from build123d import *

# Parameters (mm, degrees)
BOSS_EXTRUDE1_DEPTH = 40
FILLET1_R           = 0.5


with BuildPart() as part:
    # Sketch1 → Boss-Extrude1 (new body)
    with BuildSketch(Plane(origin=(0, 0, 0), x_dir=(-1, 0, 0), z_dir=(0, 1, 0))):
        with BuildLine():
            Line((-16.382358243, -12.416132382), (-16.309116245, 1.980717277))
            Line((-16.309116245, 1.980717277), (-2.623220974, -2.488165706))
            ThreePointArc((-2.623220974, -2.488165706), (-1.953288331, -2.586352132), (-1.288986221, -2.455382561))
            Line((-1.288986221, -2.455382561), (11.279166812, 2.343564434))
            Line((11.279166812, 2.343564434), (11.764255017, -12.063312843))
            ThreePointArc((11.764255017, -12.063312843), (11.874027832, -12.652761031), (12.15358265, -13.183183826))
            Line((12.15358265, -13.183183826), (20.699476347, -24.769483728))
            Line((20.699476347, -24.769483728), (7.033191834, -29.354905309))
            ThreePointArc((7.033191834, -29.354905309), (6.499122182, -29.629147424), (6.070505236, -30.049536105))
            Line((6.070505236, -30.049536105), (-2.58921338, -41.573541353))
            Line((-2.58921338, -41.573541353), (-10.890805488, -29.810964554))
            ThreePointArc((-10.890805488, -29.810964554), (-11.306058502, -29.378455396), (-11.830848647, -29.088464807))
            Line((-11.830848647, -29.088464807), (-25.350255054, -24.086557786))
            Line((-25.350255054, -24.086557786), (-16.834067363, -13.67200498))
            ThreePointArc((-16.834067363, -13.67200498), (-16.500364189, -13.082859401), (-16.382358243, -12.416132382))
        make_face()
    extrude(amount=BOSS_EXTRUDE1_DEPTH)

    # Fillet1
    fillet1_edges = [part.edges().sort_by_distance(p)[0] for p in [
        (18.59055185, 40, -26.587511297),
        (16.345737244, 0, -5.217707553),
        (9.46616861, 0, -0.253724215),
        (1.953288331, 0, -2.586352132),
        (-4.995090296, 0, -0.055909063),
        (-11.521710915, 0, -4.859874204),
        (-11.874027832, 0, -12.652761031),
        (11.306058502, 40, -29.378455396),
        (-16.426529498, 0, -18.976333777),
        (-13.86633409, 0, -27.062194519),
        (-6.499122182, 0, -29.629147424),
        (-1.740645928, 0, -35.811538729),
        (6.740009434, 0, -35.692252953),
        (11.306058502, 0, -29.378455396),
        (18.59055185, 0, -26.587511297),
        (21.092161209, 0, -18.879281383),
        (16.500364189, 0, -13.082859401),
        (6.740009434, 40, -35.692252953),
        (-1.740645928, 40, -35.811538729),
        (-6.499122182, 40, -29.629147424),
        (-13.86633409, 40, -27.062194519),
        (-16.426529498, 40, -18.976333777),
        (-11.874027832, 40, -12.652761031),
        (-11.521710915, 40, -4.859874204),
        (-4.995090296, 40, -0.055909063),
        (16.500364189, 40, -13.082859401),
        (1.953288331, 40, -2.586352132),
        (9.46616861, 40, -0.253724215),
        (16.345737244, 40, -5.217707553),
        (21.092161209, 40, -18.879281383),
    ]]
    fillet(fillet1_edges, radius=FILLET1_R)


solid = part.part
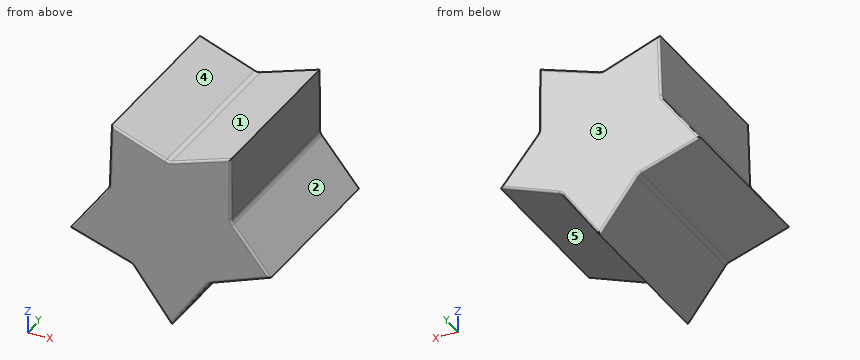
Design review of the part built by this model. Coordinates are the model's own, in mm. Face numbers are marked on the shaded views. A direction names the side the tool comes from. Round coordinates to 2 decimals unless told otherwise and drop trailing zeros. Loops run counter-clockwise (first coordinate to the right, second up) from the corner with the lowest first, then second, coordinate; pieces in that order, holes last. Notation, with made-up numbers: (40, -22) - (73, -22) arc R20 cw to (73, 2) - close; hole circle Ø9 at (76.25, 24). An arc over 180 degrees is marked (long way). One line per question, with ' | ' between items.
1. Draft analysis for pull direction X (two halves, no side actions). For the marked faces 1, 2 and 3, state which applies: released by +X, released by -X, zero draft, split by the parting line, or undercut.
Results are:
face 1: undercut | face 2: released by +X | face 3: zero draft
2. For the marked faces 4 and 5, list the 3-axis set-ups (+Z, -Z, +X, -X, +Y, -Y) from which the entire face can be reached by the end or side of a thin tool; tool diameter is ignored.
Results are:
face 4: +Z, +Y, -Y | face 5: -Z, +X, +Y, -Y
3. Clearance check with flat-ended pins moving along their axes: P1, Ø5, axis at y = 11, z = -21.5, coming from the -X side; P2, Ø8, axis at y = 35.5, z = -15, coming from the -X side; P3, Ø1.5, axis at y = 24, z = -17.5, coming from the -X side; P4, Ø2, axis at y = 7, z = -23.5, coming from the +X side. State where each tip first meets the part, or that it passes through.
Results are:
P1: stops at x = -20.13 | P2: stops at x = -16.44 | P3: stops at x = -15.89 | P4: stops at x = 25.35
4. For L1, parallel to Z at x = -18, y = 24; L2, parallel to Z at x = 8.5, y = 8; L3, parallel to X at y = 30, z = -30.5, list the stretches that pass through material, from the lowest coordinate up. Write a range as [from, to].
Results are:
L1: z = [-25.68, -21.11] | L2: z = [-33.2, -0.57] | L3: x = [-5.73, 10.4]
5. We need section A-A, the plane y = 22.5. State the section outline as (x, z) points, and give its area (3 significant figures).
Results are:
outline: (-20.7, -24.77) - (-7.03, -29.35) arc R2 cw to (-6.07, -30.05) - (2.59, -41.57) - (10.89, -29.81) arc R2 cw to (11.83, -29.09) - (25.35, -24.09) - (16.83, -13.67) arc R2 cw to (16.38, -12.42) - (16.31, 1.98) - (2.62, -2.49) arc R2 cw to (1.29, -2.46) - (-11.28, 2.34) - (-11.76, -12.06) arc R2 cw to (-12.15, -13.18) - close | area: 1,050 mm²
